from build123d import *

# Parameters (mm, degrees)
ESBO_O1_W                  = 115
ESBO_O1_H                  = 80
ESBO_O1_W_2                = 12.008486519
ESBO_O1_H_2                = 2.098343741
ESBO_O1_W_3                = 14.991513481
ESBO_O1_H_3                = 7.310170624
ESBO_O1_W_4                = 15
ESBO_O1_H_4                = 7.061661657
ESBO_O1_H_5                = 6.81374745
ESBO_O1_W_5                = 14.997964619
ESBO_O1_W_6                = 12
ESBO_O1_H_6                = 6.901670661
ESBO_O1_H_7                = 7.197630057
ESBO_O1_H_8                = 8.61677581
RESSALTO_EXTRUS_O1_DEPTH   = 6
ESBO_O2_W                  = 3
ESBO_O2_H                  = 3.99391125
ESBO_O2_H_2                = 6.002879156
CORTE_EXTRUS_O1_DEPTH      = 58.5
CORTE_EXTRUS_O1_DEPTH_BACK = 58.5


with BuildPart() as part:
    # Esboço1 → Ressalto-extrusão1 (new body)
    with BuildSketch(Plane.XY):
        with Locations((0, -0.783923472)):
            Rectangle(ESBO_O1_W, ESBO_O1_H)
        with Locations((-48.49575674, -32.734751602)):
            Rectangle(ESBO_O1_W_2, ESBO_O1_H_2, mode=Mode.SUBTRACT)
        with Locations((-29.995756741, -32.734751602)):
            Rectangle(ESBO_O1_W_3, ESBO_O1_H_2, mode=Mode.SUBTRACT)
        with Locations((-48.49575674, -25.030494419)):
            Rectangle(ESBO_O1_W_2, ESBO_O1_H_3, mode=Mode.SUBTRACT)
        with Locations((-29.995756741, -25.030494419)):
            Rectangle(ESBO_O1_W_3, ESBO_O1_H_3, mode=Mode.SUBTRACT)
        with Locations((-10, -32.734751602)):
            Rectangle(ESBO_O1_W_4, ESBO_O1_H_2, mode=Mode.SUBTRACT)
        with Locations((-10, -25.030494419)):
            Rectangle(ESBO_O1_W_4, ESBO_O1_H_3, mode=Mode.SUBTRACT)
        with Locations((-48.49575674, -14.844578279)):
            Rectangle(ESBO_O1_W_2, ESBO_O1_H_4, mode=Mode.SUBTRACT)
        with Locations((-29.995756741, -14.844578279)):
            Rectangle(ESBO_O1_W_3, ESBO_O1_H_4, mode=Mode.SUBTRACT)
        with Locations((-48.49575674, -4.906873725)):
            Rectangle(ESBO_O1_W_2, ESBO_O1_H_5, mode=Mode.SUBTRACT)
        with Locations((-29.995756741, -4.906873725)):
            Rectangle(ESBO_O1_W_3, ESBO_O1_H_5, mode=Mode.SUBTRACT)
        with Locations((-10, -14.844578279)):
            Rectangle(ESBO_O1_W_4, ESBO_O1_H_4, mode=Mode.SUBTRACT)
        with Locations((-10, -4.906873725)):
            Rectangle(ESBO_O1_W_4, ESBO_O1_H_5, mode=Mode.SUBTRACT)
        with Locations((9.99898231, -32.734751602)):
            Rectangle(ESBO_O1_W_5, ESBO_O1_H_2, mode=Mode.SUBTRACT)
        with Locations((9.99898231, -25.030494419)):
            Rectangle(ESBO_O1_W_5, ESBO_O1_H_3, mode=Mode.SUBTRACT)
        with Locations((30.00101769, -32.734751602)):
            Rectangle(ESBO_O1_W_5, ESBO_O1_H_2, mode=Mode.SUBTRACT)
        with Locations((48.5, -32.734751602)):
            Rectangle(ESBO_O1_W_6, ESBO_O1_H_2, mode=Mode.SUBTRACT)
        with Locations((30.00101769, -25.030494419)):
            Rectangle(ESBO_O1_W_5, ESBO_O1_H_3, mode=Mode.SUBTRACT)
        with Locations((48.5, -25.030494419)):
            Rectangle(ESBO_O1_W_6, ESBO_O1_H_3, mode=Mode.SUBTRACT)
        with Locations((9.99898231, -14.844578279)):
            Rectangle(ESBO_O1_W_5, ESBO_O1_H_4, mode=Mode.SUBTRACT)
        with Locations((9.99898231, -4.906873725)):
            Rectangle(ESBO_O1_W_5, ESBO_O1_H_5, mode=Mode.SUBTRACT)
        with Locations((30.00101769, -14.844578279)):
            Rectangle(ESBO_O1_W_5, ESBO_O1_H_4, mode=Mode.SUBTRACT)
        with Locations((48.5, -14.844578279)):
            Rectangle(ESBO_O1_W_6, ESBO_O1_H_4, mode=Mode.SUBTRACT)
        with Locations((30.00101769, -4.906873725)):
            Rectangle(ESBO_O1_W_5, ESBO_O1_H_5, mode=Mode.SUBTRACT)
        with Locations((48.5, -4.906873725)):
            Rectangle(ESBO_O1_W_6, ESBO_O1_H_5, mode=Mode.SUBTRACT)
        with Locations((-48.49575674, 4.950835331)):
            Rectangle(ESBO_O1_W_2, ESBO_O1_H_6, mode=Mode.SUBTRACT)
        with Locations((-29.995756741, 4.950835331)):
            Rectangle(ESBO_O1_W_3, ESBO_O1_H_6, mode=Mode.SUBTRACT)
        with Locations((-10, 4.950835331)):
            Rectangle(ESBO_O1_W_4, ESBO_O1_H_6, mode=Mode.SUBTRACT)
        with Locations((-48.49575674, 15.00048569)):
            Rectangle(ESBO_O1_W_2, ESBO_O1_H_7, mode=Mode.SUBTRACT)
        with Locations((-29.995756741, 15.00048569)):
            Rectangle(ESBO_O1_W_3, ESBO_O1_H_7, mode=Mode.SUBTRACT)
        with Locations((-48.49575674, 25.907688623)):
            Rectangle(ESBO_O1_W_2, ESBO_O1_H_8, mode=Mode.SUBTRACT)
        with Locations((-29.995756741, 25.907688623)):
            Rectangle(ESBO_O1_W_3, ESBO_O1_H_8, mode=Mode.SUBTRACT)
        with Locations((-10, 15.00048569)):
            Rectangle(ESBO_O1_W_4, ESBO_O1_H_7, mode=Mode.SUBTRACT)
        with Locations((-10, 25.907688623)):
            Rectangle(ESBO_O1_W_4, ESBO_O1_H_8, mode=Mode.SUBTRACT)
        with Locations((9.99898231, 4.950835331)):
            Rectangle(ESBO_O1_W_5, ESBO_O1_H_6, mode=Mode.SUBTRACT)
        with Locations((30.00101769, 4.950835331)):
            Rectangle(ESBO_O1_W_5, ESBO_O1_H_6, mode=Mode.SUBTRACT)
        with Locations((48.5, 4.950835331)):
            Rectangle(ESBO_O1_W_6, ESBO_O1_H_6, mode=Mode.SUBTRACT)
        with Locations((9.99898231, 15.00048569)):
            Rectangle(ESBO_O1_W_5, ESBO_O1_H_7, mode=Mode.SUBTRACT)
        with Locations((9.99898231, 25.907688623)):
            Rectangle(ESBO_O1_W_5, ESBO_O1_H_8, mode=Mode.SUBTRACT)
        with Locations((30.00101769, 15.00048569)):
            Rectangle(ESBO_O1_W_5, ESBO_O1_H_7, mode=Mode.SUBTRACT)
        with Locations((48.5, 15.00048569)):
            Rectangle(ESBO_O1_W_6, ESBO_O1_H_7, mode=Mode.SUBTRACT)
        with Locations((30.00101769, 25.907688623)):
            Rectangle(ESBO_O1_W_5, ESBO_O1_H_8, mode=Mode.SUBTRACT)
        with Locations((48.5, 25.907688623)):
            Rectangle(ESBO_O1_W_6, ESBO_O1_H_8, mode=Mode.SUBTRACT)
    extrude(amount=RESSALTO_EXTRUS_O1_DEPTH)

    # Esboço2 → Corte-extrusão1 (cut, two sides)
    with BuildSketch(Plane(origin=(0, 0, 0), x_dir=(0, 0, -1), z_dir=(1, 0, 0))) as corte_extrus_o1_sk:
        with Locations((-3, -38.786967847)):
            Rectangle(ESBO_O2_W, ESBO_O2_H)
        with Locations((-3, 36.21463695)):
            Rectangle(ESBO_O2_W, ESBO_O2_H_2)
    extrude(amount=CORTE_EXTRUS_O1_DEPTH, mode=Mode.SUBTRACT)
    extrude(corte_extrus_o1_sk.sketch, amount=-CORTE_EXTRUS_O1_DEPTH_BACK, mode=Mode.SUBTRACT)


solid = part.part
For this review, take the finished solid that the model builds, in its own axes (mm). A direction names the side the tool comes from. Coordinates: 2 decimals unless noted, no trailing zeros. Loops run counter-clockwise (first coordinate to the right, second up) from the corner with the lowest first, then second, coordinate; pieces in that order, holes last. Notation, with made-up numbers: (-17.5, 27) - (14.5, 27) arc R7 cw to (14.5, 35) - close; hole circle Ø6 at (82.25, -24.75). An arc over 180 degrees is marked (long way). Use a Markdown table: item, result. Add a question column.
Item 1: Mouldability with a two-part tool opening along X and no side actions: class faces 3 (the face through (-57.5, -1, 3)), 4 (the face through (30, -21.375, 3)), 5 (the face through (-1, 0, 0)) as pulls with the +X half, pulls with the -X half, needs draft (parallel to the pull), parting line crosses it, or undercut.
Item 2: We need section B-B (x = -0.5). Give the boundary of the cut face in (y, z).
Item 3: For line 1 (Z direction, x = 51, y = 36.5); line 2 (Y direction, x = 0, z = 2.6), list the stretches that pass through material, from the lowest coordinate up.
Item 4: We need section A-A (y = 5). Give the boundary of the cut face in (x, z), and give its area (3 significant figures).
Item 5: Tool access review of faces 1 (the face through (1, -39, 1.5)), 2 (the face through (30, -33.784, 3)): name each direction out of +Z, -Z, +X, -X, +Y, -Y from which nothing blocks a thin tool from reaching the whole face with its end or side.
Item 6: We need section C-C (z = 2.9). Give the number of separate pieces and of enclosed holes in the cut face, and give its area (3 significant figures).
Results list:
| question | item | result |
|---|---|---|
| 1 | face 3 | pulls with the -X half |
| 1 | face 4 | undercut |
| 1 | face 5 | needs draft |
| 2 | outline | (-40.78, 0) - (39.22, 0) - (39.22, 1.5) - (33.21, 1.5) - (33.21, 4.5) - (39.22, 4.5) - (39.22, 6) - (-40.78, 6) - (-40.78, 4.5) - (-36.79, 4.5) - (-36.79, 1.5) - (-40.78, 1.5) - close |
| 3 | line 1 | z = 0 to 1.5, 4.5 to 6 |
| 3 | line 2 | y = -36.79 to 33.21 |
| 4 | outline | (-57.5, 0) - (-54.5, 0) - (-54.5, 6) - (-57.5, 6) - close; (-42.49, 0) - (-37.49, 0) - (-37.49, 6) - (-42.49, 6) - close; (-22.5, 0) - (-17.5, 0) - (-17.5, 6) - (-22.5, 6) - close; (-2.5, 0) - (2.5, 0) - (2.5, 6) - (-2.5, 6) - close; (17.5, 0) - (22.5, 0) - (22.5, 6) - (17.5, 6) - close; (37.5, 0) - (42.5, 0) - (42.5, 6) - (37.5, 6) - close; (54.5, 0) - (57.5, 0) - (57.5, 6) - (54.5, 6) - close |
| 4 | area | 186 mm^2 |
| 5 | face 1 | +X, -X, -Y |
| 5 | face 2 | +Z, -Z |
| 6 | separate pieces | 1 |
| 6 | enclosed holes | 42 |
| 6 | area | 4,190 mm^2 |
